Could you check a few things on this model? Use its own coordinates, in mm. A direction names the side the tool comes from. Round coordinates to 2 decimals unless told otherwise and drop trailing zeros. Loops run counter-clockwise (first coordinate to the right, second up) from the corner with the lowest first, then second, coordinate; pieces in that order, holes last. Notation, with made-up numbers: M 14,-1 L 21,-1 A29 cw 21,25 Z; hole C -25,1.5 d2. An arc over 180 degrees is marked long. Answer in a Markdown table with one row per item.
Autodesk Inventor part; units mm, degrees
ref_plane "YZ Plane" through (0, 0, 0) normal (1, 0, 0) x (0, 1, 0)
ref_plane "XZ Plane" through (0, 0, 0) normal (0, 1, 0) x (-1, 0, 0)
ref_plane "XY Plane" through (0, 0, 0) normal (0, 0, 1) x (1, 0, 0)
sketch "Sketch1" plane through (0, 0, 0) normal (0, 0, 1) x (1, 0, 0)
  line L0 (0, 0) -> (45, 0)
  line L1 (45, 0) -> (45, 3)
  line L2 (45, 3) -> (0, 3)
  line L3 (0, 3) -> (0, 0)
  line L4 (0, 0) -> (-5.5, 0)
  line L5 (-5.5, 0) -> (-5.5, 1.5)
  line L6 (-5.5, 1.5) -> (0, 1.5)
  line L7 (0, 1.5) -> (0, 0)
  line L8 (45, 0) -> (50.5, 0)
  line L9 (50.5, 0) -> (50.5, 1.5)
  line L10 (50.5, 1.5) -> (45, 1.5)
  line L11 (45, 1.5) -> (45, 0)
  dimension "d0" = 3
  dimension "d1" = 45
  dimension "d2" = 1.5
  dimension "d3" = 5.5
  dimension "d4" = 1.5
  dimension "d5" = 5.5
revolve "Revolution1" add sketch "Sketch1" angle 360 about axis through (0, 0, 0) along (1, 0, 0)
fillet "Fillet1" radius 0.5 2 edges at (45, -1.5, 0) (0, -1.5, 0)
chamfer "Chamfer1" distance 0.5 angle 45 4 edges at (-5.5, -1.5, 0) (0, -3, 0) (45, -3, 0) (50.5, -1.5, 0)
sketch "Sketch2" plane through (0, 0, 0) normal (0, 1, 0) x (-1, 0, 0)
  line L0 (-10.2, 3) -> (-11, 3)
  line L1 (-11, 3) -> (-11, 2.85)
  line L2 (-11, 2.85) -> (-10.2, 2.85)
  line L3 (-10.2, 2.85) -> (-10.2, 3)
  line L4 (-0.5, -3) -> (-0.5, 3)
  line L5 (-44.5, 3) -> (-44.5, -3)
  line L6 (6.7, 0) -> (-40.2, 0)
  line L7 (0, 2.5) -> (0, -2.5)
  line L8 (-30.2, 3) -> (-31, 3)
  line L9 (-31, 3) -> (-31, 2.85)
  line L10 (-31, 2.85) -> (-30.2, 2.85)
  line L11 (-30.2, 2.85) -> (-30.2, 3)
  line L12 (-45, -2.5) -> (-45, 2.5)
  point P0 (0, 0)
  dimension "d11" = 2.85
  dimension "d12" = 0.8
  dimension "d15" = 0.8
  dimension "d17" = 20
  dimension "d19" = 14
  dimension "d20" = 11
revolve "Revolution2" cut sketch "Sketch2" angle 360 about axis through (-10, 0, 0) along (1, 0, 0)
equation "\"d4\" = d2"
equation "\"d15\" = d12"
properties part number "Top_Separator Shaft" material "Aluminum 6061"
1) Will these pins go through, and if not, where does the flat tip stop? P1, Ø3, axis at x = 29, y = 2, coming from the +Z side; P2, Ø1, axis at x = 43.5, z = -1, coming from the -Y side; P3, Ø1.5, axis at x = 30.5, z = -1, coming from the +Y side; P4, Ø2.5, axis at y = -1, z = 1, coming from the +X side.
Computed:
| item | result |
|---|---|
| P1 | stops at z = 2.96 |
| P2 | stops at y = -2.96 |
| P3 | stops at y = 2.98 |
| P4 | stops at x = 50.5 |
2) Which directions (+Z, -Z, +X, -X, +Y, -Y) give clear straight access to the entire face, cutting with the end or side of a thin tool? Please do faces 4 (the face through (-2.72, -1.5, 0.07)), 5 (the face through (10.594, -1.734, -2.262)), 6 (the face through (47.72, -1.5, -0.07)), 7 (the face through (20, -3, 0)).
Computed:
| item | result |
|---|---|
| face 4 | -X |
| face 5 | none |
| face 6 | +X |
| face 7 | +X, -X |
3) I want a section at A-A, the plane x = 34. Please give me the cut outline in (y, z), plus the area to 3 significant figures.
Computed:
| item | result |
|---|---|
| outline | C 0,0 d6 |
| area | 28.3 mm² |
4) I need wall thicknesses on line 1 (Y direction, x = 6, z = 0.95); line 2 (X direction, y = -1.55, z = 1.85); line 3 (X direction, y = 2.7, z = -1.2). Which ranges of each line are inside material? Lowest first, please.
Computed:
| item | result |
|---|---|
| line 1 | y = -2.85 to 2.85 |
| line 2 | x = 0 to 45 |
| line 3 | x = 0.45 to 10.2, 11 to 30.2, 31 to 44.55 |
5) If we mould it in two halves opening along X, with no side actions, what happens to faces 1 (the face through (38, -3, 0)), 2 (the face through (30.594, -1.734, -2.262)), 3 (the face through (0, -1, 2))? For each: released by +X, released by -X, zero draft, split by the parting line, or undercut.
Computed:
| item | result |
|---|---|
| face 1 | zero draft |
| face 2 | undercut |
| face 3 | released by -X |
